from build123d import *

# Parameters (mm, degrees)
BOX048_W     = 5
BOX048_H     = 58
BOX048_DEPTH = 25
FILLET053_R  = 2
BOX050_W     = 1
BOX050_H     = 62
BOX050_DEPTH = 29
FILLET055_R  = 4
BOX049_W     = 2
BOX049_H     = 60
BOX049_DEPTH = 27
FILLET054_R  = 3
FILLET056_R  = 1
FILLET057_R  = 0.99


with BuildPart() as fillet053:
    # Box048 → Box048 (new body)
    with BuildSketch(Plane(origin=(118, 56, 86), x_dir=(1, 0, 0), z_dir=(0, 0, 1))):
        with Locations((2.5, 29)):
            Rectangle(BOX048_W, BOX048_H)
    extrude(amount=BOX048_DEPTH)

    # Fillet053
    fillet053_edges = [fillet053.edges().sort_by_distance(p)[0] for p in [
        (120.5, 56, 86),
        (120.5, 56, 111),
        (120.5, 114, 86),
        (120.5, 114, 111),
    ]]
    fillet(fillet053_edges, radius=FILLET053_R)


with BuildPart() as fillet055:
    # Box050 → Box050 (new body)
    with BuildSketch(Plane(origin=(118, 54, 84), x_dir=(1, 0, 0), z_dir=(0, 0, 1))):
        with Locations((0.5, 31)):
            Rectangle(BOX050_W, BOX050_H)
    extrude(amount=BOX050_DEPTH)

    # Fillet055
    fillet055_edges = [fillet055.edges().sort_by_distance(p)[0] for p in [
        (118.5, 54, 84),
        (118.5, 54, 113),
        (118.5, 116, 84),
        (118.5, 116, 113),
    ]]
    fillet(fillet055_edges, radius=FILLET055_R)


with BuildPart() as fillet055_1:
    # Fillet055 placement: moved
    add(fillet055.part.moved(Location((4, 0, 0))))


with BuildPart() as fillet057:
    # Box049 → Box049 (new body)
    with BuildSketch(Plane(origin=(118, 55, 85), x_dir=(1, 0, 0), z_dir=(0, 0, 1))):
        with Locations((1, 30)):
            Rectangle(BOX049_W, BOX049_H)
    extrude(amount=BOX049_DEPTH)

    # Fillet054
    fillet054_edges = [fillet057.edges().sort_by_distance(p)[0] for p in [
        (119, 55, 85),
        (119, 55, 112),
        (119, 115, 85),
        (119, 115, 112),
    ]]
    fillet(fillet054_edges, radius=FILLET054_R)


with BuildPart() as fillet057_1:
    # Fillet054 placement: moved
    add(fillet057.part.moved(Location((3, 0, 0))))

    # Fusion006: union Fillet055
    add(fillet055_1.part)

    # Cut036: cut Fillet053
    add(fillet053.part, mode=Mode.SUBTRACT)

    # Fillet056
    fillet056_edges = [fillet057_1.edges().sort_by_distance(p)[0] for p in [
        (123, 85, 111),
        (123, 85, 86),
    ]]
    fillet(fillet056_edges, radius=FILLET056_R)

    # Fillet057
    fillet057_edges = [fillet057_1.edges().sort_by_distance(p)[0] for p in [
        (123, 85, 84),
        (123, 85, 113),
    ]]
    fillet(fillet057_edges, radius=FILLET057_R)


solid = fillet057_1.part
Check sheet for the modelled part. Datum: model origin and axes. Units: mm. A direction names the side the tool comes from. Give positions to 0.01 mm unless a question says otherwise; leave off trailing zeros. Loops run counter-clockwise (first coordinate to the right, second up) from the corner with the lowest first, then second, coordinate; pieces in that order, holes last. Notation, with made-up numbers: M 24.5,35 L 64.5,35 A17 ccw 64.5,47 Z; hole C 14,-9 d3. An arc over 180 degrees is marked long. Use a Markdown table: item, result. Add a question column.
Q1. Mould release check, pull along Z, two halves, no side actions. Record for faces 5 (the cylindrical face through (121.51, 56.57, 110.4)), 6 (the cylindrical face through (121.51, 55.86, 85.9)), 7 (the cylindrical face through (121.51, 114.14, 111.1)): pulls with the +Z half, pulls with the -Z half, needs draft (parallel to the pull), parting line crosses it, or undercut.
Q2. Tool access check on faces 1 (the cylindrical face through (121.51, 55.86, 111.1)), 2 (the cylindrical face through (121.51, 114.14, 85.9)), 3 (the flat face through (121, 76, 111.4)), 4 (the cylindrical face through (121.51, 113.43, 86.6)). Record the directions out of +Z, -Z, +X, -X, +Y, -Y that give a thin tool (end or side, any length) a straight path to the whole face; none if there is none.
Q3. Sectioned sample at C-C, the plane x = 121.5. Record the cut outline in (y, z), then the cut area to 3 significant figures.
Q4. Go/stop test with flat-tipped pins: pin 1 (0.8 mm diameter, centred on x = 121.5, y = 78.5, fed in from +Z); pin 2 (6 mm diameter, centred on y = 80.5, z = 90.5, fed in from +X). Record where each tip stops, or that it passes through.
Q5. Scan lines: line 1 along Z through (x, y) = (121.55, 58); line 2 along Y through (x, z) = (122.1, 106.5); line 3 along Z through (x, y) = (122.1, 102.5). Record each from-to range of solid material in increasing order. Write a range as [from, to].
Verdict:
| question | item | result |
|---|---|---|
| 1 | face 5 | undercut |
| 1 | face 6 | pulls with the -Z half |
| 1 | face 7 | pulls with the +Z half |
| 2 | face 1 | +Z, -X, -Y |
| 2 | face 2 | -Z, -X, +Y |
| 2 | face 3 | +Z, -Z, -X, +Y, -Y |
| 2 | face 4 | +X, -X |
| 3 | outline | M 55,88 A3 ccw 58,85 L 112,85 A3 ccw 115,88 L 115,109 A3 ccw 112,112 L 58,112 A3 ccw 55,109 Z; hole M 56,88 A2 ccw 58,86 L 112,86 A2 ccw 114,88 L 114,109 A2 ccw 112,111 L 58,111 A2 ccw 56,109 Z |
| 3 | area | 166 mm^2 |
| 4 | pin 1 | z = 112 |
| 4 | pin 2 | through |
| 5 | line 1 | [85, 86], [111, 112] |
| 5 | line 2 | [54, 55.99], [114.01, 116] |
| 5 | line 3 | [84, 85.99], [111.01, 113] |
